Can you work these out from the model? Positions are in its coordinate system, mm. A direction names the side the tool comes from. Coordinates: 2 decimals unless noted, no trailing zeros. Order: outer loops, then holes, each group sorted by start corner. A loop starts at its lowest first (then second) coordinate and runs counter-clockwise, first axis right, second up. Notation, with made-up numbers: (76.25, 9.25) -> (89.25, 9.25) arc R24 ccw to (89.25, 25.25) -> close; hole circle Ø8 at (-11.75, -12). An arc over 180 degrees is marked (long way). Answer as CSV lines item,"result".
from build123d import *

# Parameters (mm, degrees)
F0_W      = 2.542533
F0_H      = 2.280801
F0_R      = 0.4953
F2_DEPTH  = 6.35
F1_W      = 4.075531
F1_H      = 3.664239
F3_DEPTH  = 1.016
F3_FACE_R = 0.4953
F4_DEPTH  = 7.62


with BuildPart() as f2:
    # F0 (on Top) → F2 (new body)
    with BuildSketch(Plane.XY):
        with Locations((0.025189, 0.020531)):
            Rectangle(F0_W, F0_H)
        Circle(F0_R, mode=Mode.SUBTRACT)
    extrude(amount=-F2_DEPTH)

    # F1 (on Top) → F3 (join)
    with BuildSketch(Plane.XY):
        with Locations((-0.030896, -0.035554)):
            Rectangle(F1_W, F1_H)
    extrude(amount=-F3_DEPTH)

    # F3_face (on face) → F4 (join)
    with BuildSketch(Plane(origin=(0, 0, -1.016), x_dir=(1, 0, 0), z_dir=(0, 0, -1))):
        Circle(F3_FACE_R)
    extrude(amount=-F4_DEPTH)


solid = f2.part
Q1. Imagine slicing it at D-D (x = 0). List the corners of the cut face in (y, z) for me.
Solution:
outline,"(-1.87, -1.02) -> (-1.12, -1.02) -> (-1.12, -6.35) -> (-0.5, -6.35) -> (-0.5, -1.02) -> (0.5, -1.02) -> (0.5, -6.35) -> (1.16, -6.35) -> (1.16, -1.02) -> (1.8, -1.02) -> (1.8, 0) -> (0.5, 0) -> (0.5, 6.6) -> (-0.5, 6.6) -> (-0.5, 0) -> (-1.87, 0) -> close"
Q2. Which directions (+Z, -Z, +X, -X, +Y, -Y) give clear straight access to the entire face, cutting with the end or side of a thin tool? Please do faces 4 (the flat face through (-1.246, 0, -4)), 5 (the flat face through (1.296, 0, -4)), 6 (the cylindrical face through (-0.06, 0.49, -3.65)), 7 (the cylindrical face through (-0.06, -0.49, 3.26)).
Solution:
face 4,"-Z, -X, +Y, -Y"
face 5,"-Z, +X, +Y, -Y"
face 6,"-Z"
face 7,"+Z"
Q3. For P1, Ø1.3, axis at x = 0.5, z = -4.5, coming from the -Y side; P2, Ø1, axis at x = -1, z = -3, coming from the +Y side; P3, Ø1.8, axis at y = 0, z = -3.5, coming from the +X side, each with a flat end and sliding along its axis, tell me the tip position at first contact or that it passes through.
Solution:
P1,"y = -1.12"
P2,"y = 1.16"
P3,"x = 1.3"
Q4. Imagine slicing it at B-B (z = -2.5). List the corners of the cut face in (x, y) for me.
Solution:
outline,"(-1.25, -1.12) -> (1.3, -1.12) -> (1.3, 1.16) -> (-1.25, 1.16) -> close; hole circle Ø0.99 at (0, 0)"
Q5. Imagine slicing it at A-A (x = 0.75). List the corners of the cut face in (y, z) for me.
Solution:
outline,"(-1.87, -1.02) -> (-1.12, -1.02) -> (-1.12, -6.35) -> (1.16, -6.35) -> (1.16, -1.02) -> (1.8, -1.02) -> (1.8, 0) -> (-1.87, 0) -> close"
Q6. If I drill on line 1 (X direction, y = -0.05, z = -6); line 2 (Y direction, x = 0, z = -5.05); line 3 (Z direction, x = 1.2, y = 0.05), over which ranges is the centre line in solid material (lowest first)?
Solution:
line 1,"-1.25 to -0.49, 0.49 to 1.3"
line 2,"-1.12 to -0.5, 0.5 to 1.16"
line 3,"-6.35 to 0"
Q7. Imagine slicing it at C-C (y = 0). List the corners of the cut face in (x, z) for me.
Solution:
outline,"(-2.07, -1.02) -> (-1.25, -1.02) -> (-1.25, -6.35) -> (-0.5, -6.35) -> (-0.5, -1.02) -> (0.5, -1.02) -> (0.5, -6.35) -> (1.3, -6.35) -> (1.3, -1.02) -> (2.01, -1.02) -> (2.01, 0) -> (0.5, 0) -> (0.5, 6.6) -> (-0.5, 6.6) -> (-0.5, 0) -> (-2.07, 0) -> close"
Q8. We'd pull the mould along Y, two halves only. Please class faces 1 (the flat face through (0, 0, -1.016)), 2 (the flat face through (-2.069, -0.1, -0.5)), 3 (the flat face through (0, -1.12, -4)): pulls with the +Y half, pulls with the -Y half, needs draft (parallel to the pull), parting line crosses it, or undercut.
Solution:
face 1,"undercut"
face 2,"needs draft"
face 3,"pulls with the -Y half"
